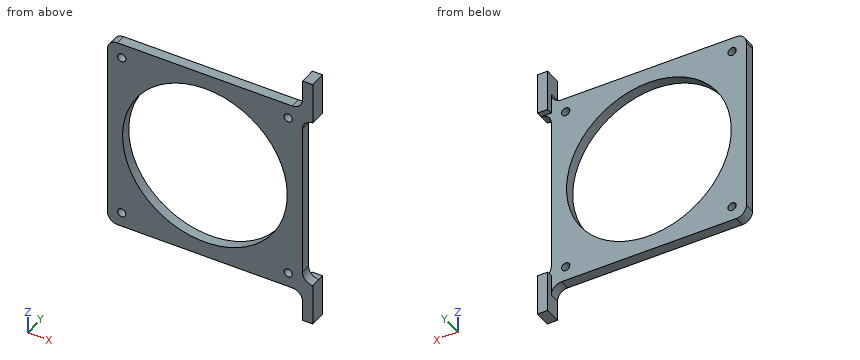
from build123d import *

# Parameters (mm, degrees)
SKETCH1_W             = 95
SKETCH1_H             = 95
SKETCH1_W_2           = 81
SKETCH1_H_2           = 81
SKETCH1_R             = 40.1
BOSS_EXTRUDE1_DEPTH   = 5
F_4_0MM_DOWEL_HOLE1_D = 4
SKETCH5_W             = 5
SKETCH5_H             = 20
BOSS_EXTRUDE2_DEPTH   = 5
SKETCH6_W             = 5
SKETCH6_H             = 20
BOSS_EXTRUDE3_DEPTH   = 3
FILLET1_R             = 5


with BuildPart() as part:
    # Sketch1 → Boss-Extrude1 (new body)
    # profile 1 of 2: a face of its own
    with BuildSketch(Plane(origin=(0, 0, 0), x_dir=(1, 0, 0), z_dir=(0, 1, 0))):
        Rectangle(SKETCH1_W, SKETCH1_H)
        Rectangle(SKETCH1_W_2, SKETCH1_H_2, mode=Mode.SUBTRACT)
    # profile 2 of 2: a face of its own
    with BuildSketch(Plane(origin=(0, 0, 0), x_dir=(1, 0, 0), z_dir=(0, 1, 0))):
        Rectangle(SKETCH1_W_2, SKETCH1_H_2)
        with Locations(Location((0, 0, 0), (0, 0, 270))):
            Circle(SKETCH1_R, mode=Mode.SUBTRACT)
    extrude(amount=BOSS_EXTRUDE1_DEPTH)

    # Ø4.0mm Dowel Hole1 (through all)
    with Locations(Plane(origin=(0, 0, 0), x_dir=(-1, 0, 0), z_dir=(0, -1, 0))):
        with Locations((40.5, -40.5), (-40.5, -40.5), (-40.5, 40.5), (40.5, 40.5)):
            Hole(F_4_0MM_DOWEL_HOLE1_D / 2)

    # Sketch5 → Boss-Extrude2 (add)
    with BuildSketch(Plane(origin=(0, 0, 0), x_dir=(1, 0, 0), z_dir=(0, 1, 0))):
        with Locations((50, -52.5)):
            Rectangle(SKETCH5_W, SKETCH5_H)
        with Locations((50, 52.5)):
            Rectangle(SKETCH5_W, SKETCH5_H)
    extrude(amount=BOSS_EXTRUDE2_DEPTH)

    # Sketch6 → Boss-Extrude3 (add)
    with BuildSketch(Plane(origin=(0, 5, 0), x_dir=(1, 0, 0), z_dir=(0, 1, 0))):
        with Locations((50, -52.5)):
            Rectangle(SKETCH6_W, SKETCH6_H)
        with Locations((50, 52.5)):
            Rectangle(SKETCH6_W, SKETCH6_H)
    extrude(amount=BOSS_EXTRUDE3_DEPTH)

    # Fillet1
    fillet1_edges = [part.edges().sort_by_distance(p)[0] for p in [
        (-47.5, 2.5, -47.5),
        (-47.5, 2.5, 47.5),
        (47.5, 2.5, 47.5),
        (47.5, 2.5, 42.5),
        (47.5, 2.5, -42.5),
        (47.5, 2.5, -47.5),
    ]]
    fillet(fillet1_edges, radius=FILLET1_R - 0.0001)  # a hair under: the kernel refuses the full size


solid = part.part
Design review of the part built by this model. Coordinates are the model's own, in mm. Coordinates: 2 decimals unless noted, no trailing zeros. Write each loop counter-clockwise with the first axis right and the second up, starting at its lowest first coordinate (ties: lowest second). Pieces come first, ordered by that corner, then holes. Notation, with made-up numbers: (18, 1.5) - (61, 1.5) arc R31 ccw to (61, 31.5) - close; hole circle Ø6 at (-31, 81.25). An arc over 180 degrees is marked (long way). One line per item, written item: value.
1) Insertion check: pin 1 (1 mm diameter, centred on x = -11, y = 4, fed in from -Z); pin 2 (3.5 mm diameter, centred on x = 40.5, z = 40.5, fed in from -Y); pin 3 (1.5 mm diameter, centred on x = -14, y = 3.5, fed in from +Z); pin 4 (4.5 mm diameter, centred on x = 40.5, z = -40.5, fed in from +Y). Each pin has a flat end and moves straight along its axis. Give the tip position at first contact, or say it passes through.
Answer sheet:
pin 1: stops at z = -47.5
pin 2: passes through
pin 3: stops at z = 47.5
pin 4: stops at y = 5
2) Add section B-B (x = 0). State the section outline as (y, z) points.
Answer sheet:
outline: (0, -47.5) - (5, -47.5) - (5, -40.1) - (0, -40.1) - close; (0, 40.1) - (5, 40.1) - (5, 47.5) - (0, 47.5) - close
3) To check wall thickness, follow probe 1 along Z at (x, y) = (-40.5, 1.4); probe 2 along X at (y, z) = (4, 0); probe 3 along X at (y, z) = (3.15, 40.5). State the ranges of each line that lie inside material, in increasing order.
Answer sheet:
probe 1: z = -47.5 to -42.5, -38.5 to 38.5, 42.5 to 47.5
probe 2: x = -47.5 to -40.1, 40.1 to 47.5
probe 3: x = -47.5 to -42.5, -38.5 to 38.5, 42.5 to 48.5
4) Add section A-A (z = 0). State the section outline as (x, y) points, plus the area to 3 significant figures.
Answer sheet:
outline: (-47.5, 0) - (-40.1, 0) - (-40.1, 5) - (-47.5, 5) - close; (40.1, 0) - (47.5, 0) - (47.5, 5) - (40.1, 5) - close
area: 74.0 mm2
